Design review of the part built by this model. Coordinates are the model's own, in mm. A direction names the side the tool comes from. Coordinates: 2 decimals unless noted, no trailing zeros. Order: outer loops, then holes, each group sorted by start corner. A loop starts at its lowest first (then second) coordinate and runs counter-clockwise, first axis right, second up.
from build123d import *

# Parameters (mm, degrees)
F0_W      = 25.4
F0_H      = 25.4
F1_DEPTH  = 12.7
F2_R      = 9.525
F3_DEPTH  = 10.16
F4_R      = 8.255
F5_DEPTH  = 2.541
F6_R      = 1.27
F7_DEPTH  = 12.701
F8_R      = 1.27
F9_DEPTH  = 12.701
F10_R     = 1.27
F11_DEPTH = 12.701
F12_R     = 1.27
F13_DEPTH = 12.701


with BuildPart() as f1:
    # F0 (on Top) → F1 (new body)
    with BuildSketch(Plane.XY):
        with Locations((12.7, 12.7)):
            Rectangle(F0_W, F0_H)
    extrude(amount=F1_DEPTH)

    # F2 (on face) → F3 (cut)
    with BuildSketch(Plane.XY.offset(12.7)):
        with Locations((12.7, 12.7)):
            Circle(F2_R)
    extrude(amount=-F3_DEPTH, mode=Mode.SUBTRACT)

    # F4 (on face) → F5 (cut, through all)
    with BuildSketch(Plane.XY.offset(2.54)):
        with Locations((12.7, 12.7)):
            Circle(F4_R)
    extrude(amount=-F5_DEPTH, mode=Mode.SUBTRACT)

    # F6 (on face) → F7 (cut, through all)
    with BuildSketch(Plane.XY.offset(12.7)):
        with Locations((2.787879, 3.091837)):
            Circle(F6_R)
    extrude(amount=-F7_DEPTH, mode=Mode.SUBTRACT)

    # F8 (on face) → F9 (cut, through all)
    with BuildSketch(Plane.XY.offset(12.7)):
        with Locations((2.428474, 23.200024)):
            Circle(F8_R)
    extrude(amount=-F9_DEPTH, mode=Mode.SUBTRACT)

    # F10 (on face) → F11 (cut, through all)
    with BuildSketch(Plane.XY.offset(12.7)):
        with Locations((22.069965, 3.077724)):
            Circle(F10_R)
    extrude(amount=-F11_DEPTH, mode=Mode.SUBTRACT)

    # F12 (on face) → F13 (cut, through all)
    with BuildSketch(Plane.XY.offset(12.7)):
        with Locations((22.441011, 22.695344)):
            Circle(F12_R)
    extrude(amount=-F13_DEPTH, mode=Mode.SUBTRACT)


solid = f1.part
1. Mouldability with a two-part tool opening along X and no side actions: class faces 1 (the flat face through (25.4, 13, 6)), 2 (the flat face through (13, 25.4, 6)), 3 (the cylindrical face through (21.062, 2.305, 6.439)) as pulls with the +X half, pulls with the -X half, needs draft (parallel to the pull), parting line crosses it, or undercut.
2. Add section D-D (z = 1). Give the boundary of the cut face in (x, y) (3 decimals).
3. Add section A-A (x = 12.7). Give the boundary of the cut face in (y, z) (3 decimals), and give its area (3 significant figures).
4. For faces 4 (the flat face through (18, 4, 12.7)), 5 (the flat face through (10, 21, 2.54)), list the 3-axis set-ups (+Z, -Z, +X, -X, +Y, -Y) from which the entire face can be reached by the end or side of a thin tool; tool diameter is ignored.
5. Add section C-C (x = 22.75). Give the boundary of the cut face in (y, z).
6. To check wall thickness, follow line 1 (Z direction, x = 3.5, y = 11); line 2 (X direction, y = 9.5, z = 10.25); line 3 (Y direction, x = 18.5, z = 3.25). State the ranges of each line that lie inside material, in increasing order.
Solution:
1. face 1: pulls with the +X half
1. face 2: needs draft
1. face 3: undercut
2. outline: (0, 0) - (25.4, 0) - (25.4, 25.4) - (0, 25.4) - close; hole circle Ø2.54 at (2.428, 23.2); hole circle Ø2.54 at (2.788, 3.092); hole circle Ø16.51 at (12.7, 12.7); hole circle Ø2.54 at (22.07, 3.078); hole circle Ø2.54 at (22.441, 22.695)
3. outline: (0, 0) - (4.445, 0) - (4.445, 2.54) - (3.175, 2.54) - (3.175, 12.7) - (0, 12.7) - close; (20.955, 0) - (25.4, 0) - (25.4, 12.7) - (22.225, 12.7) - (22.225, 2.54) - (20.955, 2.54) - close
3. area: 87.1 mm2
4. face 4: +Z, +X, -X, +Y, -Y
4. face 5: +Z
5. outline: (0, 0) - (2.01, 0) - (2.01, 12.7) - (0, 12.7) - close; (4.15, 0) - (21.46, 0) - (21.46, 12.7) - (4.15, 12.7) - close; (23.93, 0) - (25.4, 0) - (25.4, 12.7) - (23.93, 12.7) - close
6. line 1: z = 0 to 2.54
6. line 2: x = 0 to 3.73, 21.67 to 25.4
6. line 3: y = 0 to 5.14, 20.26 to 25.4
